from build123d import *

# Parameters (mm, degrees)
F0_W     = 31.75
F0_H     = 50.8
F1_DEPTH = 9.525
F2_W     = 17.78
F2_H     = 1.016
F3_DEPTH = 58.42
F4_SIZE  = 1.27
F7_DEPTH = 0.7874


with BuildPart() as f1:
    # F0 (on Top) → F1 (new body)
    with BuildSketch(Plane.XY):
        Rectangle(F0_W, F0_H)
    extrude(amount=F1_DEPTH)

    # F2 (on face) → F3 (cut)
    with BuildSketch(Plane.XZ.offset(25.4)):
        with Locations((0, 3.683)):
            Rectangle(F2_W, F2_H)
    extrude(amount=-F3_DEPTH, mode=Mode.SUBTRACT)

    # F4
    f4_edges = [f1.edges().sort_by_distance(p)[0] for p in [
        (-15.875, 0, 9.525),
        (15.875, 0, 9.525),
        (0, -25.4, 9.525),
        (0, 25.4, 9.525),
        (-15.875, -25.4, 4.7625),
        (-15.875, 25.4, 4.7625),
        (15.875, 25.4, 4.7625),
        (15.875, -25.4, 4.7625),
    ]]
    chamfer(f4_edges, length=F4_SIZE)

    # F6 (on face) → F7 (cut)
    with BuildSketch(Plane.XY.offset(9.525)):
        with BuildLine():
            add(Edge.make_bspline(
                [(-6.4422910614, -9.992572479), (-6.576387638, -9.5277504866), (-2.9682513045, -5.5271485494), (-1.6230370241, -3.3267226029), (-0.1391517651, -2.3837543589), (-3.2745475931, -1.8910386002), (-4.4465516447, -0.1797364285), (-6.7888228815, 1.3070519976), (-7.888095117, 3.0827671512), (-9.4719419101, 4.3360710627), (-10.3052427191, 5.0482783915), (-11.7938524336, 5.3782417952), (-12.4842332356, 6.5829203), (-10.32925606, 5.2604715213), (-8.8451225007, 5.3133712001), (-7.5041527627, 4.6355935651), (-5.7727147566, 5.1814768448), (-4.0784426049, 4.6283461923), (-1.9873135315, 4.0916530706), (-1.108705884, 3.7615835829), (-1.6486852677, 6.5590375218), (-1.4710237672, 8.7687761974), (-1.0661623991, 10.7075732038), (-0.0610322166, 12.855636179), (1.2394716743, 14.6101225048), (2.3332163777, 15.7965761736), (2.5641123266, 16.4961779341), (3.252212115, 15.2178296727), (3.8540014355, 13.7730672833), (4.5585807656, 12.2961361883), (4.8257092414, 10.5291786991), (5.4097550677, 9.4613192433), (5.6340869151, 7.5627733225), (5.3266594346, 6.4884408338), (4.8950565869, 5.3286938068), (5.0601967769, 4.3396482601), (5.041123295, 3.5576924459), (5.4972037108, 2.4843281805), (5.9602740046, 3.7655404276), (7.1142399283, 4.6168015862), (8.0528024254, 5.3075552814), (8.7220878624, 5.3658636167), (9.3004070886, 5.380882436), (9.765063634, 5.1626351357), (10.2212334129, 5.0276867702), (10.521522363, 4.8066763864), (10.6884480245, 4.7128941565), (11.0688814513, 4.7603953024), (11.2323128826, 4.8813015119), (11.4523118748, 4.9065218961), (11.6408865133, 4.8752991874), (11.7926899892, 4.7857749875), (11.750485731, 4.6303349314), (11.6017892672, 4.4808231583), (11.4819118772, 4.3517434996), (11.3218017, 4.1565276582), (11.0066595601, 3.657677632), (10.8380601263, 3.3525955918), (10.6583433698, 2.933851586), (10.4502325895, 2.6481420558), (10.2539582326, 2.2588087396), (9.8756355327, 1.8550879004), (9.6252045102, 1.6491392204), (9.4701910215, 1.4534911373), (9.2726879661, 1.3463737098), (9.2265213781, 0.9109138219), (9.0874966435, 0.3398509189), (8.9620205457, -0.1310281139), (8.7310528775, -0.6459707167), (8.5089153347, -1.2188165983), (8.2716856279, -1.660544323), (7.7650531821, -2.3433500022), (7.058572815, -3.0316958873), (6.2786373328, -3.3954442295), (5.4932410272, -3.9034684174), (4.9521468897, -4.0406062951), (4.5835422446, -4.0413084885), (3.9631062689, -4.5319073147), (3.4102105666, -4.5287631488), (2.7699499357, -4.6692566402), (2.0767651322, -4.7850268217), (1.4604520985, -4.8904421235), (0.8279800508, -5.0195910317), (0.4250010726, -5.0308740722), (-0.1703625544, -5.390322009), (-0.4112720451, -5.780687892), (-0.5018080947, -6.2536290481), (-0.5456870856, -6.6366625746), (-0.5362555398, -6.9175416952), (-0.6106373398, -7.3195509206), (-1.2240352375, -7.6132252976), (-1.8316007812, -8.1769049773), (-2.9486193154, -8.9853873298), (-3.9487797942, -9.4402211085), (-4.9500394796, -9.9030628486), (-5.7487292428, -10.0484224765), (-6.397083294, -10.1492771843), (-6.4422910614, -9.992572479)],
                knots=[0, 0, 0, 0, 0.0259583215, 0.0463470715, 0.0567251674, 0.0738079829, 0.0907844627, 0.1091718607, 0.1256889827, 0.1413976537, 0.1533148285, 0.1673981773, 0.17647171, 0.1915663411, 0.2062111205, 0.2194305564, 0.2340371558, 0.2494254623, 0.2662405005, 0.2741870684, 0.2914307839, 0.3091818467, 0.3248382765, 0.3421461096, 0.3591987917, 0.37359296, 0.3806487222, 0.3923027758, 0.4071889257, 0.4216976763, 0.4365182631, 0.4491655771, 0.4644212141, 0.4765478409, 0.4888771884, 0.4999804433, 0.5105377457, 0.5201314395, 0.5307861511, 0.5449434096, 0.5569882646, 0.5660330692, 0.5744812832, 0.5825287377, 0.5903862073, 0.5971191632, 0.602028747, 0.6087917991, 0.6139450483, 0.6191009197, 0.6241252147, 0.6284637057, 0.6325603162, 0.6377614234, 0.6424385646, 0.6481191834, 0.6567479492, 0.6636575486, 0.671125053, 0.6778457736, 0.6853132107, 0.6937265181, 0.7002034218, 0.7057032178, 0.7107202105, 0.7179400004, 0.7267299464, 0.7346319678, 0.7431207361, 0.7519146763, 0.7598931863, 0.7702511207, 0.7814694511, 0.7920526642, 0.8029761348, 0.8112001577, 0.8179276915, 0.8276426626, 0.836041303, 0.8451293318, 0.8546194381, 0.8636840382, 0.872611968, 0.8798430239, 0.8889941392, 0.8966487669, 0.9044270279, 0.9114121696, 0.9173799068, 0.9241469938, 0.9330649947, 0.9435250122, 0.9567341565, 0.9687796228, 0.9804435568, 0.991248712, 1, 1, 1, 1], degree=3))
        make_face()
    extrude(amount=-F7_DEPTH, mode=Mode.SUBTRACT)


solid = f1.part
CAD build for the part. Positions are in the model's coordinates, mm. A direction names the side the tool comes from. Give positions to 0.01 mm unless a question says otherwise; leave off trailing zeros. Order: outer loops, then holes, each group sorted by start corner. A loop starts at its lowest first (then second) coordinate and runs counter-clockwise, first axis right, second up. Notation, with made-up numbers: (-6.75, 25.25) -> (4.25, 25.25) arc R36 cw to (4.25, 61.25) -> close; hole circle Ø5 at (0, 83). An arc over 180 degrees is marked (long way). Return JSON: item names as keys, results as strings.
Q1. Saw through at A-A (y = -21.5). Write the cut outline in (x, z) (3 decimals), then the cut area to 3 significant figures.
Working result:
{"outline": "(-15.875, 0) -> (15.875, 0) -> (15.875, 8.255) -> (14.605, 9.525) -> (-14.605, 9.525) -> (-15.875, 8.255) -> close; hole (-8.89, 3.175) -> (8.89, 3.175) -> (8.89, 4.191) -> (-8.89, 4.191) -> close", "area": "283 mm²"}
Q2. Mould opens along X. For faces 4 (the face through (-8.89, 0, 4)), 5 (the face through (-15.231, -24.774, 4.07)), 6 (the face through (15.249, -24.756, 4.07)) say: pulls with the +X half, pulls with the -X half, needs draft (parallel to the pull), parting line crosses it, or undercut.
Working result:
{"face 4": "undercut", "face 5": "pulls with the -X half", "face 6": "pulls with the +X half"}
Q3. Flat gauge pin, fed straight in: pin 1 (9 mm diameter, centred on x = 1.5, y = 0.5, fed in from +Z) (3 decimals). Where does the tip first touch, or does it go through?
Working result:
{"pin 1": "z = 9.525"}
Q4. Drill centre lines: line 1 (Z direction, x = -1.5, y = 15.5) (3 decimals); line 2 (Z direction, x = 2.5, y = 16) (3 decimals); line 3 (X direction, y = 8, z = 4) (3 decimals). Where is each one in solid material? Low to high.
Working result:
{"line 1": "0 to 3.175, 4.191 to 9.525", "line 2": "0 to 3.175, 4.191 to 8.738", "line 3": "-15.875 to -8.89, 8.89 to 15.875"}
Q5. Which spindle directions (+Z, -Z, +X, -X, +Y, -Y) get a long thin tool onto all of the face, cutting with end or side? Do faces 1 (the face through (0, 0, 4.191)), 2 (the face through (0, 25.4, 3)), 3 (the face through (2, 2, 8.738)). Say none if no direction does.
Working result:
{"face 1": "+Y, -Y", "face 2": "+Z, -Z, +X, -X, +Y", "face 3": "+Z"}
